CAD build for the part. Positions are in the model's coordinates, mm. Face numbers are marked on the shaded views. Give positions to 0.01 mm unless a question says otherwise; leave off trailing zeros. Loops run counter-clockwise (first coordinate to the right, second up) from the corner with the lowest first, then second, coordinate; pieces in that order, holes last. Notation, with made-up numbers: M -2,-20 L 12,-20 A10 cw 12,-7 Z; hole C -37,1 d4. An arc over 180 degrees is marked long. One line per question, with ' | ' between items.
Autodesk Inventor part; units mm, degrees
ref_plane "Work Plane1" through (16.0728, 0, 0) normal (0, 0.8660254, -0.5) x (-1, 0, 0)
ref_plane "YZ Plane" through (0, 0, 0) normal (1, 0, 0) x (0, 1, 0)
ref_plane "XZ Plane" through (0, 0, 0) normal (0, 1, 0) x (-1, 0, 0)
sketch "Sketch1" plane through (0, 0, 0) normal (1, 0, 0) x (0, 1, 0)
  line L0 (5.7735, 0) -> (2.8868, -5)
  line L1 (2.8868, -5) -> (-2.8868, -5)
  line L2 (-2.8868, -5) -> (-5.7735, 0)
  line L3 (-5.7735, 0) -> (-2.8868, 5)
  line L4 (-2.8868, 5) -> (2.8868, 5)
  line L5 (2.8868, 5) -> (5.7735, 0)
  point P0 (0, 0)
  point P1 (0, 0)
  dimension "d0" = 11.547
extrude "Body" add sketch "Sketch1" along normal blind 5
sketch "Sketch2" plane through (0, 0, 0) normal (-1, 0, 0) x (0, 0, 1)
  point P0 (0, 0)
hole "Thread" at (0, 0, 0) direction (1, 0, 0) diameter 4.917 end through all
chamfer "Chamfer1" distance 0.5413 angle 30 1 edges at (0, 0, -2.4585) measured on face at (0, -3.5612, 2.1322)
chamfer "Chamfer2" distance 0.5413 angle 30 1 edges at (5, 0, -2.4585) measured on face at (5, -3.5612, 2.1322)
sketch "Sketch3" plane through (0, 0, 0) normal (0, 0, 1) x (1, 0, 0)
  line L0 (0, 5.7735) -> (5, 5.7735)
  line L1 (5, 2.8868) -> (5, 5.7735)
  line L2 (-1, 0) -> (6, 0)
  line L3 (4.5534, 5.7735) -> (5, 5)
  dimension "d3" = 10
  dimension "d4" = 30
revolve "Chamfer3" cut sketch "Sketch3" angle 360 about axis through (-10, 0, 0) along (1, 0, 0)
ref_plane "Work Plane1" through (16.0728, 0, 0) normal (0, 0.8660254, -0.5) x (-1, 0, 0)
equation "\"d0\" = 1.1547 * SW"
equation "\"d1\" = KOH"
equation "\"d13\" = -0.5 * GD1 + 0.5 * NND"
equation "\"d21\" = -0.5 * GD1 + 0.5 * NND"
equation "\"d15\" = -0.5 * GD1 + 0.5 * NND"
equation "\"d22\" = -0.5 * GD1 + 0.5 * NND"
equation "\"d3\" = SW01"
equation "\"d4\" = ANG2"
equation "\"ANG2\" = 30deg"
equation "\"NND\" = 6"
equation "\"KOH\" = 5"
equation "\"SW01\" = SW"
equation "\"GUL\" = 0.541266 * PTC"
equation "\"TOA\" = 30deg"
equation "\"PTC\" = 1"
equation "\"E0\" = 1.155 * SW"
equation "\"THREADDIA\" = 6"
equation "\"GAL\" = 0.541266 * PTC"
properties part number "JIS B 1181 - HN - class 1 - Finished - M6" material "Steel, Mild"
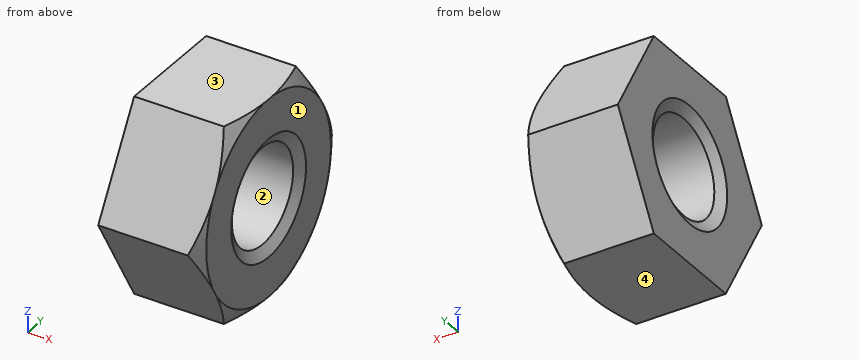
Item 1: Saw through at A-A on x = 4.15. Give the cut face in (y, z).
Conclusion:
outline: M -5.77,0 L -2.89,-5 L 2.89,-5 L 5.77,0 L 2.89,5 L -2.89,5 Z; hole C 0,0 d4.92
Item 2: Drop flat-ended pins along their axis: P1, Ø5.5, axis at y = 0, z = 0, coming from the +X side; P2, Ø3, axis at x = 1.5, z = -0.5, coming from the -Y side; P3, Ø2, axis at x = 2, y = 4.5, coming from the +Z side. Give the stop position or say it passes through.
Conclusion:
P1: x = 4.86 | P2: y = -5.77 | P3: z = 3.94
Item 3: Drill centre lines: line 1 along Z through (x, y) = (1.3, 0); line 2 along Y through (x, z) = (1.9, 0.25); line 3 along Y through (x, z) = (2.25, -1). Where is each one in solid material? Low to high. Write a range as [from, to].
Conclusion:
line 1: [-5, -2.46], [2.46, 5] | line 2: [-5.63, -2.45], [2.45, 5.63] | line 3: [-5.2, -2.25], [2.25, 5.2]
Item 4: Mould opens along Z. For the marked faces 1, 2, 3 and 4 say: pulls with the +Z half, pulls with the -Z half, needs draft (parallel to the pull), parting line crosses it, or undercut.
Conclusion:
face 1: needs draft | face 2: undercut | face 3: pulls with the +Z half | face 4: pulls with the -Z half
